```python
from build123d import *

# Parameters (mm, degrees)
SKETCH1_W               = 40
SKETCH1_H               = 94
BOSS_EXTRUDE1_DEPTH     = 2
SKETCH2_R               = 2.8
SKETCH2_W               = 21.4
SKETCH2_H               = 7.5
SKETCH2_W_2             = 8
SKETCH2_H_2             = 8
SKETCH2_W_3             = 21.1
SKETCH2_H_3             = 14.4
CUT_EXTRUDE1_DEPTH      = 52.117511677
BOSS_EXTRUDE2_DEPTH     = 21.1
BOSS_EXTRUDE3_DEPTH     = 2
SKETCH5_W               = 18.9
SKETCH5_H               = 4.55
BOSS_EXTRUDE5_DEPTH     = 2
SKETCH6_W               = 11.25
SKETCH6_H               = 19.79
BOSS_EXTRUDE6_DEPTH     = 2
SKETCH7_W               = 98.55
SKETCH7_H               = 19.79
BOSS_EXTRUDE7_DEPTH     = 2
SKETCH8_W               = 10.8
SKETCH8_H               = 19.79
SKETCH8_W_2             = 9.8
BOSS_EXTRUDE8_DEPTH     = 2
BOSS_EXTRUDE9_DEPTH     = 2
SKETCH12_R              = 1.1
CUT_EXTRUDE2_DEPTH      = 71.070582986
LPATTERN1_COUNT         = 3
LPATTERN1_PITCH         = 35
SKETCH13_W              = 25.1
SKETCH13_H              = 26.79
CUT_EXTRUDE3_DEPTH      = 2.5
FILLET1_R               = 4
FILLET2_R               = 5
CHAMFER1_SIZE           = 1
CUT_EXTRUDE4_DEPTH      = 0.5
CUT_EXTRUDE5_DEPTH      = 60.439436404
CUT_EXTRUDE5_DEPTH_BACK = 60.439436404
SKETCH15_W              = 44
SKETCH15_H              = 16.505


with BuildPart() as part:
    # Sketch1 → Boss-Extrude1 (new body)
    with BuildSketch(Plane(origin=(0, 0, 0), x_dir=(1, 0, 0), z_dir=(0, 1, 0))):
        Rectangle(SKETCH1_W, SKETCH1_H)
    extrude(amount=BOSS_EXTRUDE1_DEPTH)

    # Sketch2 → Cut-Extrude1 (cut, through all)
    with BuildSketch(Plane(origin=(0, 2, 0), x_dir=(1, 0, 0), z_dir=(0, 1, 0))):
        with Locations(Location((14.8, 40.4, 0), (0, 0, 270))):
            Circle(SKETCH2_R)
        with Locations((-0.5, 43.25)):
            Rectangle(SKETCH2_W, SKETCH2_H)
        with Locations((0.05, -20.02)):
            Rectangle(SKETCH2_W_2, SKETCH2_H_2)
        with Locations((14.05, -20.02)):
            Rectangle(SKETCH2_W_2, SKETCH2_H_2)
        with Locations((-13.95, -20.02)):
            Rectangle(SKETCH2_W_2, SKETCH2_H_2)
        with Locations((-13.95, -38.42)):
            Rectangle(SKETCH2_W_2, SKETCH2_H_2)
        with Locations((9.45, -39.8)):
            Rectangle(SKETCH2_W_3, SKETCH2_H_3)
    extrude(amount=-CUT_EXTRUDE1_DEPTH, mode=Mode.SUBTRACT)

    # Sketch3 → Boss-Extrude2 (add)
    with BuildSketch(Plane(origin=(20, 0, 0), x_dir=(0, 0, -1), z_dir=(1, 0, 0))):
        Polygon((-32.6, 2), (-34.6, 7), (-49.35, 7), (-49.35, 7.5), (-51.55, 7.5), (-51.55, 9), (-33.4, 9), (-30.6, 2), align=None)
    extrude(amount=-BOSS_EXTRUDE2_DEPTH)

    # Sketch4 → Boss-Extrude3 (add)
    with BuildSketch(Plane.ZY.offset(1.1)):
        Polygon((51.55, 9), (51.55, 2), (30.6, 2), (33.4, 9), align=None)
    extrude(amount=BOSS_EXTRUDE3_DEPTH)

    # Sketch5 → Boss-Extrude5 (add)
    with BuildSketch(Plane(origin=(0, 2, 0), x_dir=(1, 0, 0), z_dir=(0, 1, 0))):
        with Locations((-10.55, -49.275)):
            Rectangle(SKETCH5_W, SKETCH5_H)
    extrude(amount=-BOSS_EXTRUDE5_DEPTH)

    # Sketch6 → Boss-Extrude6 (add)
    with BuildSketch(Plane.XY.offset(51.55)):
        with Locations((-14.375, -7.895)):
            Rectangle(SKETCH6_W, SKETCH6_H)
    extrude(amount=-BOSS_EXTRUDE6_DEPTH)

    # Sketch7 → Boss-Extrude7 (add)
    with BuildSketch(Plane.ZY.offset(20)):
        with Locations((2.275, -7.895)):
            Rectangle(SKETCH7_W, SKETCH7_H)
    extrude(amount=BOSS_EXTRUDE7_DEPTH)

    # Sketch8 → Boss-Extrude8 (add)
    with BuildSketch(Plane(origin=(0, 0, -47), x_dir=(-1, 0, 0), z_dir=(0, 0, -1))):
        with Locations((16.6, -7.895)):
            Rectangle(SKETCH8_W, SKETCH8_H)
        with Locations((-15.1, -7.895)):
            Rectangle(SKETCH8_W_2, SKETCH8_H)
    extrude(amount=BOSS_EXTRUDE8_DEPTH)

    # Sketch9 → Boss-Extrude9 (add)
    with BuildSketch(Plane(origin=(20, 0, 0), x_dir=(0, 0, -1), z_dir=(1, 0, 0))):
        Polygon((-51.55, 9), (-51.55, -17.79), (49, -17.79), (49, 2), (-30.6, 2), (-33.4, 9), align=None)
    extrude(amount=BOSS_EXTRUDE9_DEPTH)

    # Sketch12 → Cut-Extrude2 (cut, symmetric)
    with BuildSketch(Plane(origin=(22, 0, 0), x_dir=(0, 0, -1), z_dir=(1, 0, 0))):
        with Locations((34.95, -14.79)):
            Circle(SKETCH12_R)
    cut_extrude2 = extrude(amount=CUT_EXTRUDE2_DEPTH, both=True, mode=Mode.SUBTRACT)

    # LPattern1: Cut-Extrude2 ×3
    with Locations(*[(0, 0, i * LPATTERN1_PITCH) for i in range(1, LPATTERN1_COUNT)]):
        add(cut_extrude2, mode=Mode.SUBTRACT)

    # Sketch13 → Cut-Extrude3 (cut)
    with BuildSketch(Plane.XY.offset(51.55)):
        with Locations((9.45, -4.395)):
            Rectangle(SKETCH13_W, SKETCH13_H)
    extrude(amount=-CUT_EXTRUDE3_DEPTH, mode=Mode.SUBTRACT)

    # Fillet1
    # the kernel refuses this fillet: 4 mm, written as the material it takes off along each edge
    with BuildSketch(Plane(origin=(22, -27.79, -49), x_dir=(-1, 0, 0), z_dir=(0, 1, 0))) as fillet1_piece_1:
        with BuildLine():
            CenterArc((FILLET1_R, FILLET1_R), FILLET1_R, 180, 90)
            Line((0, FILLET1_R), (0, 0))
            Line((0, 0), (FILLET1_R, 0))
        make_face()
    extrude(amount=39.79, mode=Mode.SUBTRACT)
    with BuildSketch(Plane(origin=(22, 9, 23.4), x_dir=(0, -1, 0), z_dir=(0, 0, 1))) as fillet1_piece_2:
        with BuildLine():
            CenterArc((FILLET1_R, -FILLET1_R), FILLET1_R, 90, 90)
            Line((0, -FILLET1_R), (0, 0))
            Line((0, 0), (FILLET1_R, 0))
        make_face()
    extrude(amount=35.65, mode=Mode.SUBTRACT)
    with BuildSketch(Plane(origin=(22, 2, -59), x_dir=(-1, 0, 0), z_dir=(0, 0, 1))) as fillet1_piece_3_section:
        with BuildLine():
            CenterArc((FILLET1_R, FILLET1_R), FILLET1_R, 180, 90)
            Line((0, FILLET1_R), (0, 0))
            Line((0, 0), (FILLET1_R, 0))
        make_face()
    fillet1_piece_3 = extrude(amount=99.6, mode=Mode.PRIVATE)
    fillet1_piece_3 = split(fillet1_piece_3, bisect_by=Plane(origin=(22, -28.896551724, 18.24137931), z_dir=(0, 0.3713906763541048, -0.928476690885259)), keep=Keep.TOP, mode=Mode.PRIVATE)
    add(fillet1_piece_3, mode=Mode.SUBTRACT)
    with BuildSketch(Plane(origin=(-22, -27.79, -49), x_dir=(1, 0, 0), z_dir=(0, 1, 0)), Plane(origin=(-22, 12, 51.55), x_dir=(1, 0, 0), z_dir=(0, -1, 0))) as fillet1_piece_4:
        with BuildLine():
            CenterArc((FILLET1_R, -FILLET1_R), FILLET1_R, 90, 90)
            Line((0, -FILLET1_R), (0, 0))
            Line((0, 0), (FILLET1_R, 0))
        make_face()
    extrude(amount=39.79, mode=Mode.SUBTRACT)
    with BuildSketch(Plane(origin=(-22, 2, -59), x_dir=(1, 0, 0), z_dir=(0, 0, 1))) as fillet1_piece_5:
        with BuildLine():
            CenterArc((FILLET1_R, -FILLET1_R), FILLET1_R, 90, 90)
            Line((0, -FILLET1_R), (0, 0))
            Line((0, 0), (FILLET1_R, 0))
        make_face()
    extrude(amount=120.55, mode=Mode.SUBTRACT)
    with BuildSketch(Plane(origin=(-3.1, 9, 23.4), x_dir=(0, -1, 0), z_dir=(0, 0, 1))) as fillet1_piece_6:
        with BuildLine():
            CenterArc((FILLET1_R, FILLET1_R), FILLET1_R, 180, 90)
            Line((0, FILLET1_R), (0, 0))
            Line((0, 0), (FILLET1_R, 0))
        make_face()
    extrude(amount=35.65, mode=Mode.SUBTRACT)
    with BuildSketch(Plane(origin=(22, -27.79, 49.05), x_dir=(-1, 0, 0), z_dir=(0, 1, 0))) as fillet1_piece_7:
        with BuildLine():
            CenterArc((FILLET1_R, -FILLET1_R), FILLET1_R, 90, 90)
            Line((0, -FILLET1_R), (0, 0))
            Line((0, 0), (FILLET1_R, 0))
        make_face()
    extrude(amount=46.79, mode=Mode.SUBTRACT)

    # Fillet2
    # the kernel refuses this fillet: 5 mm, written as the material it takes off along each edge
    with BuildSketch(Plane(origin=(20, 0, 32.6), x_dir=(0, 0, -1), z_dir=(-1, 0, 0))) as fillet2_piece_1:
        with BuildLine():
            CenterArc((4, -5), FILLET2_R, 90, 53.130102354)
            Line((0, -2), (0, 0))
            Line((0, 0), (4, 0))
        make_face()
    extrude(amount=21.1, mode=Mode.SUBTRACT)

    # Chamfer1
    # the kernel refuses this chamfer: 1 mm, written as the material it takes off along each edge
    with BuildSketch(Plane(origin=(-1.1, 7, 49.05), x_dir=(-1, 0, 0), z_dir=(0, -1, 0))) as chamfer1_piece_1:
        Polygon((CHAMFER1_SIZE, 0), (0, CHAMFER1_SIZE), (0, 0), align=None)
    extrude(amount=9.571682988, mode=Mode.SUBTRACT)
    with BuildSketch(Plane(origin=(-1.1, 7, 49.05), x_dir=(0, 1, 0), z_dir=(1, 0, 0))) as chamfer1_piece_2:
        Polygon((CHAMFER1_SIZE, 0), (0, -CHAMFER1_SIZE), (0, 0), align=None)
    extrude(amount=19.1, mode=Mode.SUBTRACT)
    with BuildSketch(Plane(origin=(18, 7, 45.05), x_dir=(0.919398394096703, 0, 0.3933275898438904), z_dir=(0.3933275898438904, 0, -0.919398394096703))) as chamfer1_piece_3_section:
        Polygon((4, -CHAMFER1_SIZE), (4 - CHAMFER1_SIZE, 0), (4, 0), align=None)
    chamfer1_piece_3 = revolve(axis=Axis((18, 7, 45.05), (0, -1, 0)), revolution_arc=66.838289129, mode=Mode.PRIVATE)
    chamfer1_piece_3 = split(chamfer1_piece_3, bisect_by=Plane(origin=(20, 7, 45.05), z_dir=(-1, 0, 0)), keep=Keep.TOP, mode=Mode.PRIVATE)
    add(chamfer1_piece_3, mode=Mode.SUBTRACT)
    with BuildSketch(Plane(origin=(-3.671682988, 7, 49.05), x_dir=(0, 1, 0), z_dir=(1, 0, 0))) as chamfer1_piece_4a_section:
        Polygon((CHAMFER1_SIZE, 0), (0, -CHAMFER1_SIZE), (0, 0), align=None)
    chamfer1_piece_4a = extrude(amount=21.671682988, mode=Mode.PRIVATE)
    chamfer1_piece_4a = split(chamfer1_piece_4a, bisect_by=Plane(origin=(-1.1, 7, 49.05), z_dir=(-1, 0, 0)), keep=Keep.TOP, mode=Mode.PRIVATE)
    with BuildSketch(Plane(origin=(-1.1, 9.571682988, 49.05), x_dir=(-1, 0, 0), z_dir=(0, -1, 0))) as chamfer1_piece_4b_section:
        Polygon((CHAMFER1_SIZE, 0), (0, CHAMFER1_SIZE), (0, 0), align=None)
    chamfer1_piece_4b = extrude(amount=12.143365976, mode=Mode.PRIVATE)
    chamfer1_piece_4b = split(chamfer1_piece_4b, bisect_by=Plane(origin=(-1.1, 7, 49.05), z_dir=(0, 1, 0)), keep=Keep.TOP, mode=Mode.PRIVATE)
    chamfer1_piece_4 = chamfer1_piece_4a & chamfer1_piece_4b
    add(chamfer1_piece_4, mode=Mode.SUBTRACT)

    # Sketch14 → Cut-Extrude4 (cut)
    with BuildSketch(Plane.ZY.offset(-20)):
        Polygon((47.286067977, 7), (34.6, 7), (32.6, 2), (32.6, -9.79), (47.286067977, -9.79), align=None)
    extrude(amount=-CUT_EXTRUDE4_DEPTH, mode=Mode.SUBTRACT)

    # Sketch15 → Cut-Extrude5 (cut, two sides: drawn at the far end of the back side and taken through both)
    with BuildSketch(Plane(origin=(0, 2, 0), x_dir=(1, 0, 0), z_dir=(0, 1, 0)).offset(-CUT_EXTRUDE5_DEPTH_BACK)):
        with Locations((0, -20.02)):
            Rectangle(SKETCH15_W, SKETCH15_H)
    extrude(amount=CUT_EXTRUDE5_DEPTH + CUT_EXTRUDE5_DEPTH_BACK, mode=Mode.SUBTRACT)


with BuildPart() as cut_extrude5_piece_1:
    # of the separate pieces the step leaves, piece 1, a body of its own (cut_extrude5_pieces)
    add(part.part.solids().sort_by_distance((-11.2, 2, -39.5))[0])


with BuildPart() as cut_extrude5_piece_2:
    # of the separate pieces the step leaves, piece 2, a body of its own (cut_extrude5_pieces)
    add(part.part.solids().sort_by_distance((-20, 0, 49.55))[0])


with BuildPart() as cut_extrude5_piece_2_1:
    # Body-Move/Copy1: read off the stored shape, not the designer's step
    # Body-Move/Copy1: moved
    add(cut_extrude5_piece_2.part.moved(Location((0, 0, -16.505))))

    # Combine1: union Cut-Extrude5 piece 1
    add(cut_extrude5_piece_1.part)


solid = cut_extrude5_piece_2_1.part
```
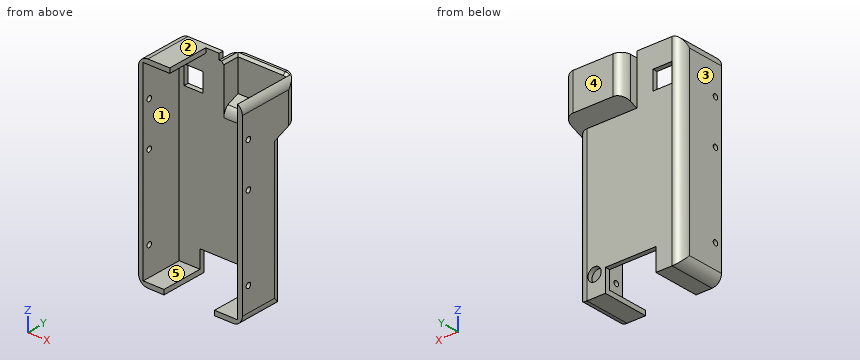
CAD build for the part. Positions are in the model's coordinates, mm. Face numbers are marked on the shaded views. A direction names the side the tool comes from. Give positions to 0.01 mm unless a question says otherwise; leave off trailing zeros. Order: outer loops, then holes, each group sorted by start corner. A loop starts at its lowest first (then second) coordinate and runs counter-clockwise, first axis right, second up. Notation, with made-up numbers: M 40.5,15.25 L 81.5,15.25 A27 ccw 81.5,40.25 Z; hole C 67.25,34 d5. An arc over 180 degrees is marked long. Put each result on its own line as item: value. Start each with the question number.
(1) Flat gauge pins, fed straight in: pin 1 Ø12 at (x, z) = (4, -19.5) entering from -Y; pin 2 Ø4 at (x, z) = (11.5, 26) entering from -Y; pin 3 Ø4 at (x, z) = (-14, -19) entering from +Y. Where does each tip first touch, or does it go through?
(2) Saw through at A-A, the plane y = -11. Write the cut outline in (x, z) (3 decimals), then the cut area to 3 significant figures.
(3) Drill centre lines: line 1 along X through (y, z) = (-5.5, -31.5); line 2 along Y through (x, z) = (-12, 26); line 3 along Y through (x, z) = (-20.8, -34.95). Where is each one in solid material? Low to high.
(4) Saw through at D-D, the plane x = 4. Write the cut outline in (y, z) (3 decimals), then the cut area to 3 significant figures.
(5) Which spindle directions (+Z, -Z, +X, -X, +Y, -Y) get a long thin tool onto all of the face, cutting with end or side? Do the marked faces 4 and 5. Say none if no direction does.
(6) Saw through at B-B, the plane z = -40.4. Write the cut outline in (x, y).
(7) Mould opens along X. For the marked faces 1, 2 and 3 say: +X half, -X half, draft (parallel to the pull), parting line (faces both ways), or undercut.
(8) Saw through at C-C, the plane x = 14.8. Write the cut outline in (y, z) (3 decimals).
Check result:
1. pin 1: stops at y = 0
1. pin 2: stops at y = 7
1. pin 3: stops at y = 2
2. outline: M -22,-45 A4 ccw -18,-49 L -11.2,-49 L -11.2,-47 L -20,-47 L -20,33.045 L -8.75,33.045 L -8.75,35.045 L -18,35.045 A4 ccw -22,31.045 Z; M 10.2,-49 L 18,-49 A4 ccw 22,-45 L 22,28.545 A4 ccw 20,32.009 L 20,-47 L 10.2,-47 Z
2. area: 377 mm2
3. line 1: x = -22 to -20, 20 to 22
3. line 2: y = 0 to 2
3. line 3: y = -17.79 to -15.89, -13.69 to 0.86
4. outline: M 0,-39.5 L 2,-39.5 L 2,14.095 L 9,16.895 L 9,32.545 L 8,32.545 L 7,31.545 L 7,18.095 L 2,16.095 A5 ccw 0,12.095 Z
4. area: 150 mm2
5. face 4: +Z, -Z, +X, -X, +Y
5. face 5: -Y
6. outline: M -22,-17.79 L -20,-17.79 L -20,0 L -11.2,0 L -11.2,2 L -18,2 A4 ccw -22,-2 Z; M 10.2,0 L 12,0 L 12,2 L 10.2,2 Z; M 17.6,0 L 20,0 L 20,-17.79 L 22,-17.79 L 22,-2 A4 ccw 18,2 L 17.6,2 Z
7. face 1: undercut
7. face 2: draft
7. face 3: -X half
8. outline: M -17.79,-49 L 2,-49 L 2,-43.2 L 0,-43.2 L 0,-47 L -17.79,-47 Z; M 0,-37.6 L 2,-37.6 L 2,14.095 L 9,16.895 L 9,32.545 L 8,32.545 L 7,31.545 L 7,18.095 L 2,16.095 A5 ccw 0,12.095 Z
